Could you check a few things on this model? Use its own coordinates, in mm. Face numbers are marked on the shaded views. A direction names the side the tool comes from. Round coordinates to 2 decimals unless told otherwise and drop trailing zeros. Write each loop counter-clockwise with the first axis right and the second up, starting at its lowest first coordinate (ties: lowest second). Pieces come first, ordered by that corner, then holes.
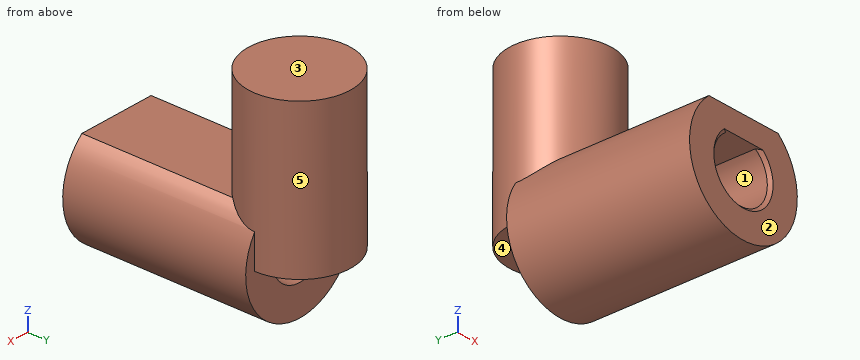
```python
from build123d import *

# Parameters (mm, degrees)
F2_DEPTH = 25.4
F3_DEPTH = 127
F4_SIZE  = 2.54
F0_R     = 42.2975618679
F5_DEPTH = 127


with BuildPart() as f2:
    # F1 (on Front) → F2 (new body)
    with BuildSketch(Plane.XZ):
        with BuildLine():
            ThreePointArc((-32.5502825036, 39.0015270077), (-0.1096585285, -50.7998816436), (32.7183586862, 38.8606356726))
            Line((32.7183586862, 38.8606356726), (-32.5502825036, 39.0015270077))
        make_face()
        with BuildLine():
            Line((-13.8090135631, 21.3183288373), (14.0783311513, 21.141442524))
            ThreePointArc((14.0783311513, 21.141442524), (-0.1611061228, -25.3994890661), (-13.8090135631, 21.3183288373))
        make_face(mode=Mode.SUBTRACT)
    extrude(amount=F2_DEPTH)

    # F3 (add): a face of the model
    f3_faces = [f2.faces().sort_by_distance(p)[0] for p in [
        (-0.1067314616, -25.4, -49.443902714),
    ]]
    extrude(f3_faces, amount=F3_DEPTH)

    # F4
    f4_edges = [f2.edges().sort_by_distance(p)[0] for p in [
        (-0.161106, -152.4, -25.399489),
    ]]
    chamfer(f4_edges, length=F4_SIZE)

    # F0 (on Top) → F5 (join)
    with BuildSketch(Plane.XY):
        Circle(F0_R)
    extrude(amount=F5_DEPTH)


solid = f2.part
```
Q1. Imagine slicing it at C-C, the plane y = -50. Write out the boundary of the cut face in (x, z).
Q2. On a 3-axis mill with a long thin cutter (end or side, diameter ignored), from which of +Z, -Z, +X, -X, +Y, -Y can I reach the whole of each face in a straight line? I mean the marked faces 1 and 2. Say none if no direction works.
Q3. I'm going to push flat-ended pins straight in: pin 1 Ø2 at (x, z) = (13, 81) entering from +Y; pin 2 Ø3 at (y, z) = (-91, -25.5) entering from -X; pin 3 Ø4 at (x, y) = (-37, -68.5) entering from +Z. Where does each tip first touch, or does it pass through?
Q4. We'd pull the mould along Z, two halves only. Please class the marked faces 3, 4 and 5: pulls with the +Z half, pulls with the -Z half, needs draft (parallel to the pull), parting line crosses it, or undercut.
Q5. Imagine slicing it at A-A, the plane x = 0. Write out the boundary of the cut face in (y, z).
Q6. Imagine slicing it at B-B, the plane z = 57. Write out the boundary of the cut face in (x, y), then the cut area to 3 significant figures.
Q7. If I drill on L1, parallel to X at y = -73, z = 0; L2, parallel to Y at x = 2, z = 79; L3, parallel to Z at x = -21, y = 20, over which ranges is the centre line in solid material (lowest first)?
Results found:
1. outline: (-32.55, 39) arc R50.8 ccw (long way) to (32.72, 38.86) - close; hole (-13.81, 21.32) arc R25.4 ccw (long way) to (14.08, 21.14) - close
2. face 1: -Y
2. face 2: +Z, -Z, +X, -X, -Y
3. pin 1: stops at y = 40.56
3. pin 2: stops at x = -44.77
3. pin 3: stops at z = 36.82
4. face 3: pulls with the +Z half
4. face 4: undercut
4. face 5: needs draft
5. outline: (-152.4, -50.8) - (0, -50.8) - (0, -25.4) - (-149.86, -25.4) - (-152.4, -27.94) - close; (-152.4, 21.23) - (-42.3, 21.23) - (-42.3, 0) - (42.3, 0) - (42.3, 127) - (-42.3, 127) - (-42.3, 38.93) - (-152.4, 38.93) - close
6. outline: circle Ø84.6 at (0, 0)
6. area: 5,620 mm2
7. L1: x = -50.8 to -25.4, 25.4 to 50.8
7. L2: y = -42.25 to 42.25
7. L3: z = 0 to 127
